from build123d import *

# Parameters (mm, degrees)
SKETCH1_R           = 6.025
BOSS_EXTRUDE1_DEPTH = 10
SKETCH3_R           = 6.025
BOSS_EXTRUDE2_DEPTH = 16.5
SKETCH5_R           = 11
BOSS_EXTRUDE3_DEPTH = 2
SKETCH6_R           = 3.3
CUT_EXTRUDE3_DEPTH  = 29.5


with BuildPart() as part:
    # Sketch1 → Boss-Extrude1 (new body)
    with BuildSketch(Plane.XY):
        Circle(SKETCH1_R)
    extrude(amount=BOSS_EXTRUDE1_DEPTH)

    # Sketch3 → Boss-Extrude2 (add)
    with BuildSketch(Plane.XY.offset(10)):
        Circle(SKETCH3_R)
    extrude(amount=BOSS_EXTRUDE2_DEPTH)

    # Sketch5 → Boss-Extrude3 (add)
    with BuildSketch(Plane(origin=(0, 0, 0), x_dir=(-1, 0, 0), z_dir=(0, 0, -1))):
        Circle(SKETCH5_R)
    extrude(amount=BOSS_EXTRUDE3_DEPTH)

    # Sketch6 → Cut-Extrude3 (cut, through all)
    with BuildSketch(Plane.XY.offset(26.5)):
        Circle(SKETCH6_R)
    extrude(amount=-CUT_EXTRUDE3_DEPTH, mode=Mode.SUBTRACT)


solid = part.part
For this review, take the finished solid that the model builds, in its own axes (mm). A direction names the side the tool comes from. Round coordinates to 2 decimals unless told otherwise and drop trailing zeros. Loops run counter-clockwise (first coordinate to the right, second up) from the corner with the lowest first, then second, coordinate; pieces in that order, holes last. Notation, with made-up numbers: (47.5, 4.25) - (89.5, 4.25) arc R13 cw to (89.5, 8.25) - close; hole circle Ø10 at (-23, 86). An arc over 180 degrees is marked (long way). Use one line per item in the form item = value.
Item 1: Consider section D-D on y = 5.5. Write out the cut boundary in (x, z), then the cut area to 3 significant figures.
Answers:
outline = (-9.53, -2) - (9.53, -2) - (9.53, 0) - (2.46, 0) - (2.46, 26.5) - (-2.46, 26.5) - (-2.46, 0) - (-9.53, 0) - close
area = 168 mm^2
Item 2: Tool access review of faces 4 (the cylindrical face through (-4.44, 4.07, 13.06)), 5 (the flat face through (3, -2, -2)): name each direction out of +Z, -Z, +X, -X, +Y, -Y from which nothing blocks a thin tool from reaching the whole face with its end or side.
Answers:
face_4 = +Z
face_5 = -Z, +X, -X, +Y, -Y
Item 3: For line 1 (Y direction, x = 0, z = 15) (3 decimals); line 2 (Z direction, x = -7.5, y = 1.5); line 3 (X direction, y = 0.5, z = 8), list the stretches that pass through material, from the lowest coordinate up.
Answers:
line_1 = -6.025 to -3.3, 3.3 to 6.025
line_2 = -2 to 0
line_3 = -6 to -3.26, 3.26 to 6
Item 4: Clearance check with flat-ended pins moving along their axes: P1, Ø12, axis at y = -8.5, z = 10, coming from the -X side; P2, Ø1.5, axis at y = 1, z = 19, coming from the +X side; P3, Ø3, axis at y = 4.5, z = 2.5, coming from the +X side (3 decimals). State where each tip first meets the part, or that it passes through.
Answers:
P1 = -5.48
P2 = 6.02
P3 = 5.225
Item 5: Consider section C-C on z = 8.75. Write out the cut boundary in (x, y) (3 decimals), then the cut area to 3 significant figures.
Answers:
outline = circle Ø12.05 at (0, 0); hole circle Ø6.6 at (0, 0)
area = 79.8 mm^2
Item 6: Consider section A-A on x = 0. Write out the cut boundary in (y, z) (3 decimals).
Answers:
outline = (-11, -2) - (-3.3, -2) - (-3.3, 26.5) - (-6.025, 26.5) - (-6.025, 0) - (-11, 0) - close; (3.3, -2) - (11, -2) - (11, 0) - (6.025, 0) - (6.025, 26.5) - (3.3, 26.5) - close
Item 7: Mouldability with a two-part tool opening along X and no side actions: class faces 1 (the flat face through (-5, -5, 0)), 2 (the cylindrical face through (-2.43, 2.23, 12.45)), 3 (the cylindrical face through (2.38, -10.74, -0.99)) as +X half, -X half, draft (parallel to the pull), parting line (faces both ways), or undercut.
Answers:
face_1 = draft
face_2 = undercut
face_3 = parting line
